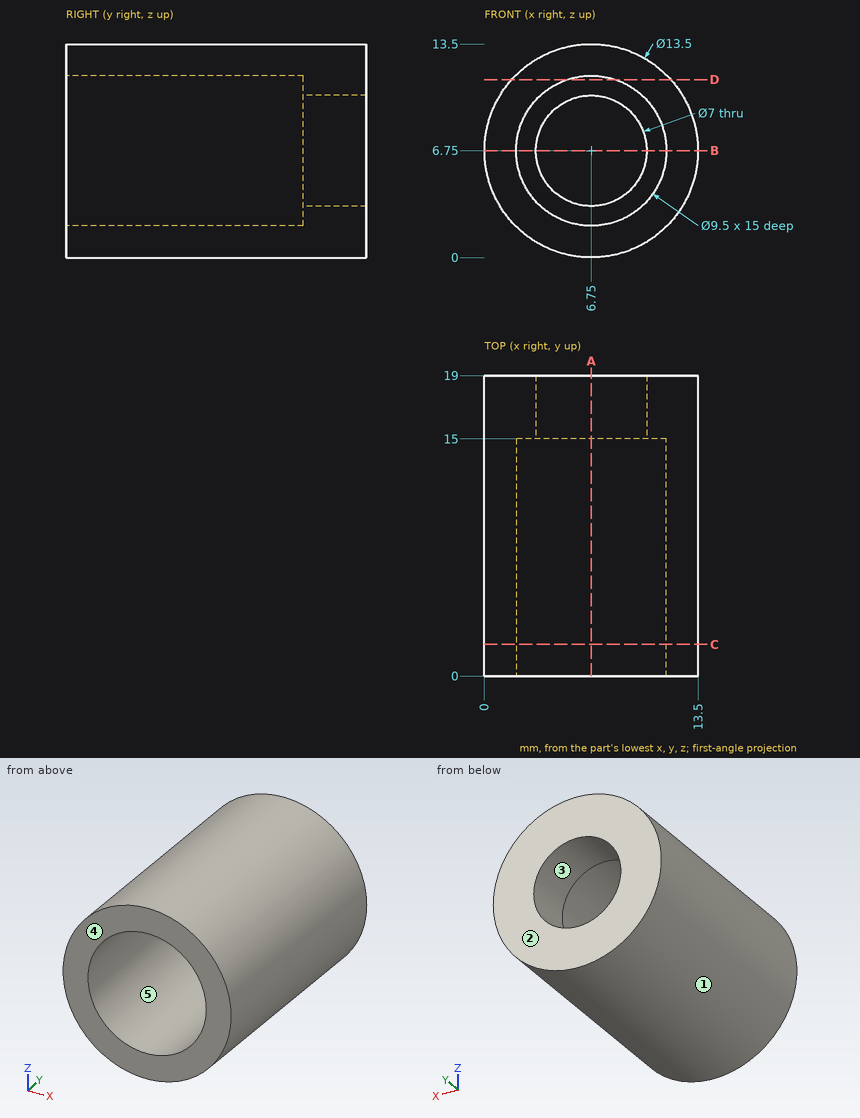
Answer from the drawing. Dimensions are ordinates in mm from the lowest x, y and z of the part. A direction names the side the tool comes from. Give positions to 0.01 mm unless a question says otherwise; leave off trailing zeros. Order: outer loops, then holes, each group sorted by start corner. A loop starts at its lowest first (then second) coordinate and runs counter-clockwise, first axis right, second up.
(1) Find section B-B (z = 6.75). Give the vertices of the cut face in (x, y), plus the area to 3 significant figures.
(2) Find section C-C (y = 2). Give the vertices of the cut face in (x, z), plus the area to 3 significant figures.
(3) Given pin 1 (6 mm diameter, centred on x = 5.5, y = 14.5, fed in from +Z); pin 2 (1.5 mm diameter, centred on y = 15, z = 11.5, fed in from +X); pin 3 (3 mm diameter, centred on x = 8.5, z = 9, fed in from -Y); pin 4 (5 mm diameter, centred on y = 7.5, z = 1.5, fed in from -X), each flat-ended and moving along its own axis, determine where each tip first touches the part or whether it passes through.
(4) Straight lines are drawn through the part: L1, parallel to Z at x = 6.75, y = 16.65; L2, parallel to Z at x = 6.75, y = 10.75. For each, find the intervals that lie inside material, in ascending order.
(5) Find section A-A (x = 6.75). Give the vertices of the cut face in (y, z).
(6) For a pull along X with two mould halves and no side action, classify the marked faces 1, 2 and 3 as released by +X, released by -X, zero draft, split by the parting line, or undercut.
(7) For the marked faces 4 and 5, determine the directions among +Z, -Z, +X, -X, +Y, -Y from which every point of the face is accessible in a straight line to the end or side of a thin tool.
(8) Find section D-D (z = 11.25). Give the vertices of the cut face in (x, y).
Result sheet:
1. outline: (0, 0) - (2, 0) - (2, 15) - (3.25, 15) - (3.25, 19) - (0, 19) - close; (10.25, 15) - (11.5, 15) - (11.5, 0) - (13.5, 0) - (13.5, 19) - (10.25, 19) - close
1. area: 86.0 mm2
2. outline: circle Ø13.5 at (6.75, 6.75); hole circle Ø9.5 at (6.75, 6.75)
2. area: 72.3 mm2
3. pin 1: stops at z = 13.5
3. pin 2: stops at x = 12.19
3. pin 3: stops at y = 15
3. pin 4: stops at x = 0.59
4. L1: z = 0 to 3.25, 10.25 to 13.5
4. L2: z = 0 to 2, 11.5 to 13.5
5. outline: (0, 0) - (19, 0) - (19, 3.25) - (15, 3.25) - (15, 2) - (0, 2) - close; (0, 11.5) - (15, 11.5) - (15, 10.25) - (19, 10.25) - (19, 13.5) - (0, 13.5) - close
6. face 1: split by the parting line
6. face 2: zero draft
6. face 3: undercut
7. face 4: +Z, -Z, +X, -X, -Y
7. face 5: -Y
8. outline: (1.72, 0) - (5.23, 0) - (5.23, 15) - (8.27, 15) - (8.27, 0) - (11.78, 0) - (11.78, 19) - (1.72, 19) - close
